Autodesk Inventor part; units mm, degrees
ref_plane "YZ Plane" through (0, 0, 0) normal (1, 0, 0) x (0, 1, 0)
ref_plane "XZ Plane" through (0, 0, 0) normal (0, 1, 0) x (-1, 0, 0)
ref_plane "XY Plane" through (0, 0, 0) normal (0, 0, 1) x (1, 0, 0)
sketch "Sketch1" plane through (0, 0, 0) normal (0, 0, 1) x (1, 0, 0)
  line L0 (-12.5, 0) -> (12.5, 0)
  line L1 (12.5, 0) -> (12.5, -80)
  line L2 (12.5, -80) -> (-12.5, -80)
  line L3 (-12.5, -80) -> (-12.5, 0)
  point P0 (0, 0)
  point P1 (0, 0)
  dimension "d0" = 25
  dimension "d1" = 80
extrude "Plate1" add sketch "Sketch1" along normal blind 2
sketch "Sketch8" plane through (0, 0, 2) normal (0, 0, 1) x (1, 0, 0)
  line L0 (-12.5, -80) -> (-12.5, 0) construction
  line L1 (12.5, -80) -> (-12.5, -80)
  line L2 (12.5, 0) -> (12.5, -80)
  line L3 (-12.5, 0) -> (12.5, 0)
  circle A0 centre (0, -70) radius 2.5
  circle A1 centre (0, -10) radius 2.5
  line L4 (-12.5, 0) -> (-12.5, -80) construction
  line L5 (-12.5, -40) -> (12.5, -40) construction
  point P0 (0, 0)
  dimension "d34" = 5
  dimension "d35" = 10
extrude "Extrusion3" cut sketch "Sketch8" against normal through all
fillet "Fillet2" radius 2 4 edges at (-12.5, -80, 1) (12.5, -80, 1) (12.5, 0, 1) (-12.5, 0, 1)
equation "\"d2\" = Thickness"
equation "\"BendReliefWidth\" = Thickness"
equation "\"BendReliefDepth\" = 0.5 * Thickness"
equation "\"CornerReliefSize\" = 4 * Thickness"
equation "\"MinimumRemnant\" = 2 * Thickness"
equation "\"TransitionRadius\" = BendRadius"
equation "\"JacobiRadiusSize\" = BendRadius"
equation "\"GapSize\" = Thickness"
properties part number "NDM 11.025 bracket 25" material "Stainless Steel"
Source: CAD feature listing. Evaluate the final solid. Frame: model axes, mm. Round coordinates to 2 decimals unless told otherwise and drop trailing zeros. Write each loop counter-clockwise with the first axis right and the second up, starting at its lowest first coordinate (ties: lowest second). Pieces come first, ordered by that corner, then holes. Notation, with made-up numbers: (68.5, 10) - (107.5, 10) arc R17 ccw to (107.5, 27) - close; hole circle Ø7 at (-18.5, 11). An arc over 180 degrees is marked (long way). Use CSV: the item, a comma, the result in double quotes. Start each with the question number.
(1) Cut plane B-B, the plane y = -70. Return loops of the section in (x, z), and give its area (3 significant figures).
(2) Cut plane A-A, the plane x = 0. Return loops of the section in (y, z).
(3) Cut plane C-C, the plane z = 0.8. Return loops of the section in (x, y).
(4) Material intervals for probe 1 along Y at (x, z) = (0, 1.35); probe 2 along Y at (x, z) = (-1.5, 1.3); probe 3 along Y at (x, z) = (-10.75, 1), sorted ascending. Write a range as [from, to].
(5) Mould query, pull axis Y, two halves, no side actions, for faces 1 (the face through (12.5, -39, 1)), 2 (the face through (-0.54, -12.44, 1.01)), 3 (the face through (0, -80, 1)), 4 (the face through (11.93, -0.6, 1.01)). Classes: pulls with the +Y half, pulls with the -Y half, needs draft (parallel to the pull), parting line crosses it, or undercut.
Geometry says:
1,outline,"(-12.5, 0) - (-2.5, 0) - (-2.5, 2) - (-12.5, 2) - close; (2.5, 0) - (12.5, 0) - (12.5, 2) - (2.5, 2) - close"
1,area,"40.0 mm²"
2,outline,"(-80, 0) - (-72.5, 0) - (-72.5, 2) - (-80, 2) - close; (-67.5, 0) - (-12.5, 0) - (-12.5, 2) - (-67.5, 2) - close; (-7.5, 0) - (0, 0) - (0, 2) - (-7.5, 2) - close"
3,outline,"(-12.5, -78) arc R2 ccw to (-10.5, -80) - (10.5, -80) arc R2 ccw to (12.5, -78) - (12.5, -2) arc R2 ccw to (10.5, 0) - (-10.5, 0) arc R2 ccw to (-12.5, -2) - close; hole circle Ø5 at (0, -70); hole circle Ø5 at (0, -10)"
4,probe 1,"[-80, -72.5], [-67.5, -12.5], [-7.5, 0]"
4,probe 2,"[-80, -72], [-68, -12], [-8, 0]"
4,probe 3,"[-79.98, -0.02]"
5,face 1,"needs draft"
5,face 2,"undercut"
5,face 3,"pulls with the -Y half"
5,face 4,"pulls with the +Y half"
